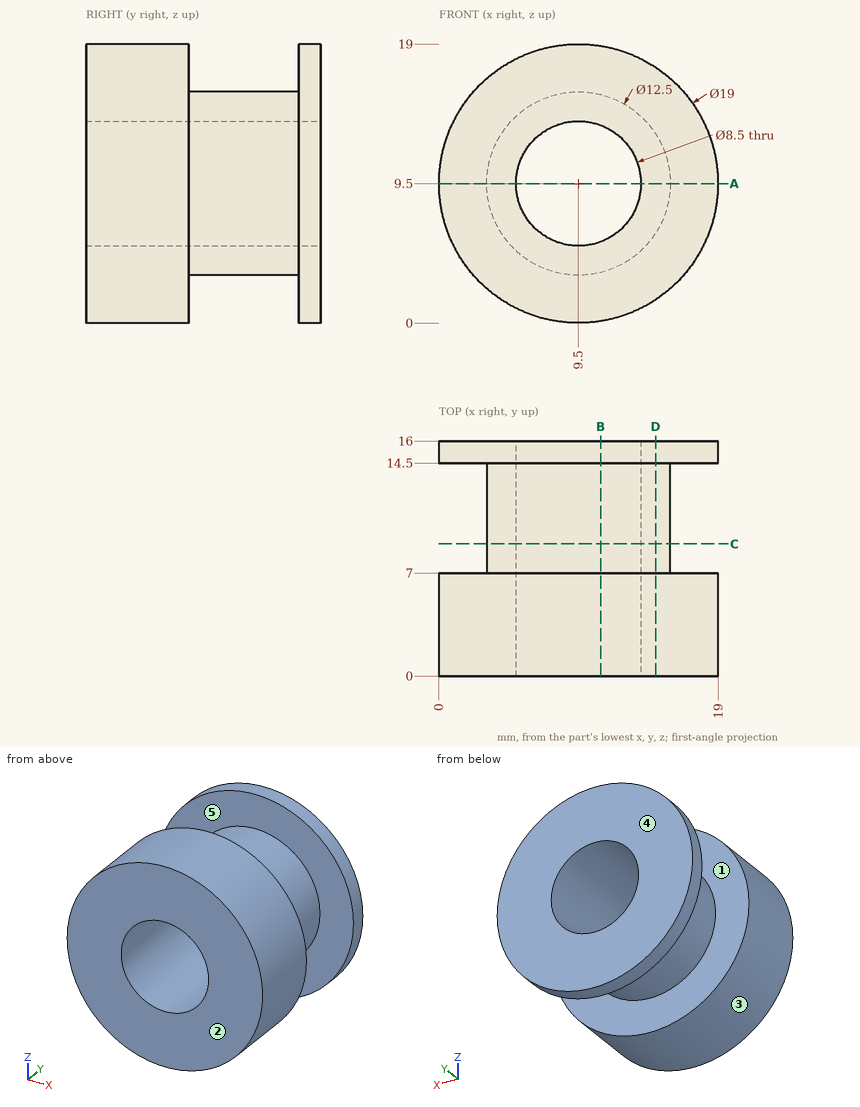
Print and shaded views of the part. All mm, measured from the part's lowest x, y and z. A direction names the side the tool comes from. Round coordinates to 2 decimals unless told otherwise and drop trailing zeros. Write each loop counter-clockwise with the first axis right and the second up, starting at its lowest first coordinate (ties: lowest second). Pieces come first, ordered by that corner, then holes. Notation, with made-up numbers: (-34, -26.5) -> (3, -26.5) arc R16 ccw to (3, -0.5) -> close; hole circle Ø1 at (49.5, 59.25). An arc over 180 degrees is marked (long way). Return JSON: item names as keys, results as strings. Group by question number.
Q1. Pin check, flat tips, straight feed: pin 1 (2 mm diameter, centred on y = 4.5, z = 5, fed in from -X); pin 2 (6 mm diameter, centred on y = 6.5, z = 14.5, fed in from +X); pin 3 (2 mm diameter, centred on y = 6, z = 13, fed in from -X). Stop position of each tip, or through.
Q2. Mould opens along Y. For the marked faces 1, 2 and 3 say: pulls with the +Y half, pulls with the -Y half, needs draft (parallel to the pull), parting line crosses it, or undercut.
Q3. Saw through at B-B on x = 11. Write the cut outline in (y, z).
Q4. Saw through at C-C on y = 9. Write the cut outline in (x, z).
Q5. Probe L1, parallel to X at y = 5.75, z = 9.5; L2, parallel to Z at x = 9.5, y = 9.25. List the from-to ranges inside material, lowest first. Write a range as [from, to].
Q6. Which spindle directions (+Z, -Z, +X, -X, +Y, -Y) get a long thin tool onto all of the face, cutting with end or side? Do the marked faces 4 and 5. Say none if no direction does.
Q7. Saw through at D-D on x = 14.75. Write the cut outline in (y, z), plus the area to 3 significant figures.
Q8. Saw through at A-A on z = 9.5. Write the cut outline in (x, y).
Answer:
{
 "1": {"pin 1": "x = 0.67", "pin 2": "x = 18.79", "pin 3": "x = 0.33"},
 "2": {"face 1": "undercut", "face 2": "pulls with the -Y half", "face 3": "needs draft"},
 "3": {"outline": "(0, 0.12) -> (7, 0.12) -> (7, 3.43) -> (14.5, 3.43) -> (14.5, 0.12) -> (16, 0.12) -> (16, 5.52) -> (0, 5.52) -> close; (0, 13.48) -> (16, 13.48) -> (16, 18.88) -> (14.5, 18.88) -> (14.5, 15.57) -> (7, 15.57) -> (7, 18.88) -> (0, 18.88) -> close"},
 "4": {"outline": "circle Ø12.5 at (9.5, 9.5); hole circle Ø8.5 at (9.5, 9.5)"},
 "5": {"L1": "[0, 5.25], [13.75, 19]", "L2": "[3.25, 5.25], [13.75, 15.75]"},
 "6": {"face 4": "+Z, -Z, +X, -X, +Y", "face 5": "none"},
 "7": {"outline": "(0, 1.58) -> (7, 1.58) -> (7, 6.11) -> (14.5, 6.11) -> (14.5, 1.58) -> (16, 1.58) -> (16, 17.42) -> (14.5, 17.42) -> (14.5, 12.89) -> (7, 12.89) -> (7, 17.42) -> (0, 17.42) -> close", "area": "185 mm2"},
 "8": {"outline": "(0, 0) -> (5.25, 0) -> (5.25, 16) -> (0, 16) -> (0, 14.5) -> (3.25, 14.5) -> (3.25, 7) -> (0, 7) -> close; (13.75, 0) -> (19, 0) -> (19, 7) -> (15.75, 7) -> (15.75, 14.5) -> (19, 14.5) -> (19, 16) -> (13.75, 16) -> close"}
}
